Autodesk Inventor part; units mm, degrees
ref_plane "YZ Plane" through (0, 0, 0) normal (1, 0, 0) x (0, 1, 0)
ref_plane "XZ Plane" through (0, 0, 0) normal (0, 1, 0) x (-1, 0, 0)
ref_plane "XY Plane" through (0, 0, 0) normal (0, 0, 1) x (1, 0, 0)
sketch "Sketch1" plane through (0, 0, 0) normal (0, 0, 1) x (1, 0, 0)
  line L0 (0, 0) -> (20, 0)
  line L1 (20, 0) -> (20, 16)
  line L2 (20, 16) -> (0, 16)
  line L3 (0, 16) -> (0, 0)
  dimension "d0" = 20
  dimension "d1" = 16
extrude "Extrusion1" add sketch "Sketch1" along normal blind 11.5
sketch "Sketch2" plane through (0, 0, 11.5) normal (0, 0, 1) x (1, 0, 0)
  line L0 (20, 0) -> (20, 16)
  line L1 (0, 0) -> (20, 0)
  point P0 (15.5, 8)
  dimension "d4" = 4.5
  dimension "d5" = 8
hole "Hole1" at (15.5, 8, 11.5) direction (0, 0, -1) diameter 4.917 end through all
sketch "Sketch3" plane through (0, 0, 0) normal (0, -1, 0) x (1, 0, 0)
  arc A0 (5.5953, 3.25) -> (5.5953, 4.75) centre (8.5, 4) ccw
  line L0 (0, 0) -> (20, 0)
  line L1 (20, 0) -> (20, 11.5)
  line L2 (0, 0) -> (0, 11.5)
  line L3 (0, 4.75) -> (5.5953, 4.75)
  line L4 (0, 3.25) -> (5.5953, 3.25)
  dimension "d13" = 4
  dimension "d14" = 11.5
  dimension "d15" = 3
  dimension "d16" = 0.75
  dimension "d17" = 0.75
extrude "Extrusion2" cut sketch "Sketch3" against normal through all
sketch "Sketch4" plane through (0, 0, 0) normal (0, -1, 0) x (1, 0, 0)
  line L0 (0, 0) -> (20, 0)
  line L1 (20, 0) -> (20, 11.5)
  point P0 (16.5, 4.8)
  point P1 (18, 2)
  dimension "d20" = 4.8
  dimension "d21" = 3.5
  dimension "d22" = 2
  dimension "d23" = 2
hole "Hole2" at (16.5, 0, 4.8) direction (0, 1, 0) diameter 2.459 depth 3.5 tip angle 118
hole "Hole3" at (18, 0, 2) direction (0, 1, 0) diameter 1.5 depth 4.5 tip angle 118
hole "Hole4" at (18, 0, 2) direction (0, 1, 0) diameter 2 depth 2 tip angle 118
sketch "Sketch5" plane through (0, 0, 11.5) normal (0, 0, 1) x (1, 0, 0)
  line L0 (0, 0) -> (20, 0)
  line L1 (20, 0) -> (20, 16)
  point P0 (2.5, 8)
  dimension "d45" = 8
  dimension "d46" = 17.5
hole "Hole5" at (2.5, 8, 11.5) direction (0, 0, -1) diameter 2.459 end up to surface
sketch "Sketch6" plane through (0, 0, 0) normal (0, 0, -1) x (-1, 0, 0)
  circle A0 centre (-2.5, 8) radius 1.2295
  point P0 (0, 0)
hole "Hole6" at (2.5, 8, 0) direction (0, 0, 1) diameter 3 end up to surface
chamfer "Chamfer1" distance 0.25 angle 45 14 edges at (0, 8, 11.5) (0, 16, 8.125) (0, 16, 1.625) (0, 8, 0) (0, 0, 1.625) (0, 0, 8.125) (10, 0, 11.5) (10, 0, 0) (20, 0, 5.75) (20, 8, 11.5) (10, 16, 11.5) (20, 8, 0) (20, 16, 5.75) (10, 16, 0)
equation "\"d17\" = d16"
properties part number "Heat Block" material "Aluminum 6061"
Verification items for the finished model (mm, model axes). A direction names the side the tool comes from. Coordinates: 2 decimals unless noted, no trailing zeros. Write each loop counter-clockwise with the first axis right and the second up, starting at its lowest first coordinate (ties: lowest second). Pieces come first, ordered by that corner, then holes. Notation, with made-up numbers: M -26,-9.75 L -11,-9.75 A21 ccw -11,0.25 Z; hole C 22.25,-14.5 d5. An arc over 180 degrees is marked long. Use a Markdown table: item, result.
Q1. Go/stop test with flat-tipped pins: P1, Ø3, axis at x = 15.5, y = 8, coming from the -Z side; P2, Ø2, axis at x = 16.5, z = 4.8, coming from the -Y side. Record where each tip stops, or that it passes through.
Reply:
| item | result |
|---|---|
| P1 | passes through |
| P2 | stops at y = 3.64 |
Q2. Thickness scan on line 1 (X direction, y = 8, z = 0.7); line 2 (X direction, y = 8, z = 9.75); line 3 (Z direction, x = 4, y = 1.75). Record the ranges inside material, lowest first.
Reply:
| item | result |
|---|---|
| line 1 | x = 0 to 1, 4 to 13.04, 17.96 to 20 |
| line 2 | x = 0 to 1.27, 3.73 to 13.04, 17.96 to 20 |
| line 3 | z = 0 to 3.25, 4.75 to 11.5 |
Q3. Sectioned sample at B-B, the plane y = 10. Record the boundary of the cut face in (x, z).
Reply:
| item | result |
|---|---|
| outline | M 0,0.25 L 0.25,0 L 14.07,0 L 14.07,11.5 L 0.25,11.5 L 0,11.25 L 0,4.75 L 5.6,4.75 A3 cw long 5.6,3.25 L 0,3.25 Z; M 16.93,0 L 19.75,0 L 20,0.25 L 20,11.25 L 19.75,11.5 L 16.93,11.5 Z |
Q4. Sectioned sample at C-C, the plane x = 2.5. Record the boundary of the cut face in (y, z).
Reply:
| item | result |
|---|---|
| outline | M 0,0.25 L 0.25,0 L 6.5,0 L 6.5,3.25 L 0,3.25 Z; M 0,4.75 L 6.77,4.75 L 6.77,11.5 L 0.25,11.5 L 0,11.25 Z; M 9.23,4.75 L 16,4.75 L 16,11.25 L 15.75,11.5 L 9.23,11.5 Z; M 9.5,0 L 15.75,0 L 16,0.25 L 16,3.25 L 9.5,3.25 Z |
Q5. Draft check along Y on faces 1 (the face through (2.131, 6.827, 8.078)), 2 (the face through (10, 0, 7)), 3 (the face through (13.062, 8.32, 5.67)), 4 (the face through (10, 8, 0)). Enter one of: +Y half, -Y half, draft (parallel to the pull), parting line (faces both ways), or undercut.
Reply:
| item | result |
|---|---|
| face 1 | undercut |
| face 2 | -Y half |
| face 3 | undercut |
| face 4 | draft |
Q6. Sectioned sample at A-A, the plane x = 8.5. Record the boundary of the cut face in (y, z).
Reply:
| item | result |
|---|---|
| outline | M 0,0.25 L 0.25,0 L 15.75,0 L 16,0.25 L 16,1 L 0,1 Z; M 0,7 L 16,7 L 16,11.25 L 15.75,11.5 L 0.25,11.5 L 0,11.25 Z |
Q7. Sectioned sample at D-D, the plane z = 10. Record the boundary of the cut face in (x, y), plus the area to 3 significant figures.
Reply:
| item | result |
|---|---|
| outline | M 0,0.25 L 0.25,0 L 19.75,0 L 20,0.25 L 20,15.75 L 19.75,16 L 0.25,16 L 0,15.75 Z; hole C 2.5,8 d2.46; hole C 15.5,8 d4.92 |
| area | 296 mm² |
Q8. Set-up check for faces 5 (the face through (4, 8, 4.75)), 6 (the face through (18.732, 3.342, 2.163)), 7 (the face through (10, 8, 11.5)), 8 (the face through (1.49, 6.89, 1.65)): record each of +Z, -Z, +X, -X, +Y, -Y from which the full face is reachable in a straight line by a thin tool's end or side.
Reply:
| item | result |
|---|---|
| face 5 | -X, +Y, -Y |
| face 6 | -Y |
| face 7 | +Z, +X, -X, +Y, -Y |
| face 8 | -Z |
